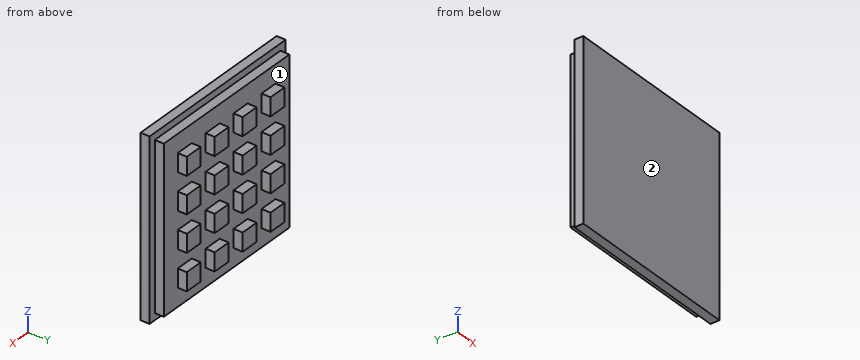
from build123d import *

# Parameters (mm, degrees)
SKETCH1_W           = 65
SKETCH1_H           = 65
BOSS_EXTRUDE1_DEPTH = 3.3
SKETCH2_W           = 60
SKETCH2_H           = 60
BOSS_EXTRUDE2_DEPTH = 3.3
SKETCH3_W           = 6.666666666
SKETCH3_H           = 6.666666666
SKETCH3_W_2         = 6.666666667
BOSS_EXTRUDE3_DEPTH = 3.3
LPATTERN1_COUNT     = 4
LPATTERN1_PITCH     = 13.3333334


with BuildPart() as part:
    # Sketch1 → Boss-Extrude1 (new body)
    with BuildSketch(Plane(origin=(0, 0, 0), x_dir=(1, 0, 0), z_dir=(0, 1, 0))):
        with Locations((32.5, 32.5)):
            Rectangle(SKETCH1_W, SKETCH1_H)
    extrude(amount=BOSS_EXTRUDE1_DEPTH)

    # Sketch2 → Boss-Extrude2 (add)
    with BuildSketch(Plane(origin=(0, 3.3, 0), x_dir=(1, 0, 0), z_dir=(0, 1, 0))):
        with Locations((32.5, 32.5)):
            Rectangle(SKETCH2_W, SKETCH2_H)
    extrude(amount=BOSS_EXTRUDE2_DEPTH)

    # Sketch3 → Boss-Extrude3 (add)
    with BuildSketch(Plane(origin=(0, 6.6, 0), x_dir=(1, 0, 0), z_dir=(0, 1, 0))):
        with Locations((12.5, 52.5)):
            Rectangle(SKETCH3_W, SKETCH3_H)
        with Locations((25.833333334, 52.5)):
            Rectangle(SKETCH3_W_2, SKETCH3_H)
        with Locations((39.166666666, 52.5)):
            Rectangle(SKETCH3_W_2, SKETCH3_H)
        with Locations((52.5, 52.5)):
            Rectangle(SKETCH3_W, SKETCH3_H)
    boss_extrude3 = extrude(amount=BOSS_EXTRUDE3_DEPTH)

    # LPattern1: Boss-Extrude3 ×4
    with Locations(*[(0, 0, i * LPATTERN1_PITCH) for i in range(1, LPATTERN1_COUNT)]):
        add(boss_extrude3)


solid = part.part
Geometry check sheet. Reference: the model listing, model coordinates, mm. Face numbers are marked on the shaded views. Coordinates: 2 decimals unless noted, no trailing zeros. Order: outer loops, then holes, each group sorted by start corner. A loop starts at its lowest first (then second) coordinate and runs counter-clockwise, first axis right, second up. Notation, with made-up numbers: (-20, 78) - (-8, 78) arc R11 ccw to (-8, 89) - close; hole circle Ø2 at (36, 5). An arc over 180 degrees is marked (long way). Answer in a Markdown table with one row per item. Add a question column.
1) Cross-section at A-A, the plane x = 61.5. Record the cut outline in (y, z), then the cut area to 4 significant figures.
2) Release check for a two-part mould opening along X. For the marked faces 1 and 2 record: +X half, -X half, draft (parallel to the pull), parting line (faces both ways), or undercut.
3) Cross-section at C-C, the plane z = -33. Record the cut outline in (x, y).
4) Cross-section at D-D, the plane y = 4.5. Record the cut outline in (x, z), then the cut area to 3 significant figures.
5) Material ranges on line 1 along Z through (x, y) = (11, 7.5); line 2 along X through (y, z) = (7.5, -12); line 3 along Y through (x, z) = (10.5, -6.5), recorded low to high. Write a range as [from, to].
6) Gauge pin test, flat ends, axial feed: P1, Ø3.5, axis at y = 8.5, z = -53, coming from the -X side; P2, Ø1.5, axis at y = 7.5, z = -36.5, coming from the +X side; P3, Ø3.5, axis at x = 53.5, y = 9, coming from the -Z side. Record the tip position at first contact, or that the pin passes through.
7) Cross-section at B-B, the plane y = 8. State how many separate pieces and enclosed holes the cut face has, then the cut area to 3 significant figures.
Check result:
| question | item | result |
|---|---|---|
| 1 | outline | (0, -65) - (3.3, -65) - (3.3, -62.5) - (6.6, -62.5) - (6.6, -2.5) - (3.3, -2.5) - (3.3, 0) - (0, 0) - close |
| 1 | area | 412.5 mm² |
| 2 | face 1 | undercut |
| 2 | face 2 | draft |
| 3 | outline | (0, 0) - (65, 0) - (65, 3.3) - (62.5, 3.3) - (62.5, 6.6) - (2.5, 6.6) - (2.5, 3.3) - (0, 3.3) - close |
| 4 | outline | (2.5, -62.5) - (62.5, -62.5) - (62.5, -2.5) - (2.5, -2.5) - close |
| 4 | area | 3,600 mm² |
| 5 | line 1 | z = [-55.83, -49.17], [-42.5, -35.83], [-29.17, -22.5], [-15.83, -9.17] |
| 5 | line 2 | x = [9.17, 15.83], [22.5, 29.17], [35.83, 42.5], [49.17, 55.83] |
| 5 | line 3 | y = [0, 6.6] |
| 6 | P1 | stops at x = 9.17 |
| 6 | P2 | stops at x = 55.83 |
| 6 | P3 | stops at z = -55.83 |
| 7 | separate pieces | 16 |
| 7 | enclosed holes | 0 |
| 7 | area | 711 mm² |
